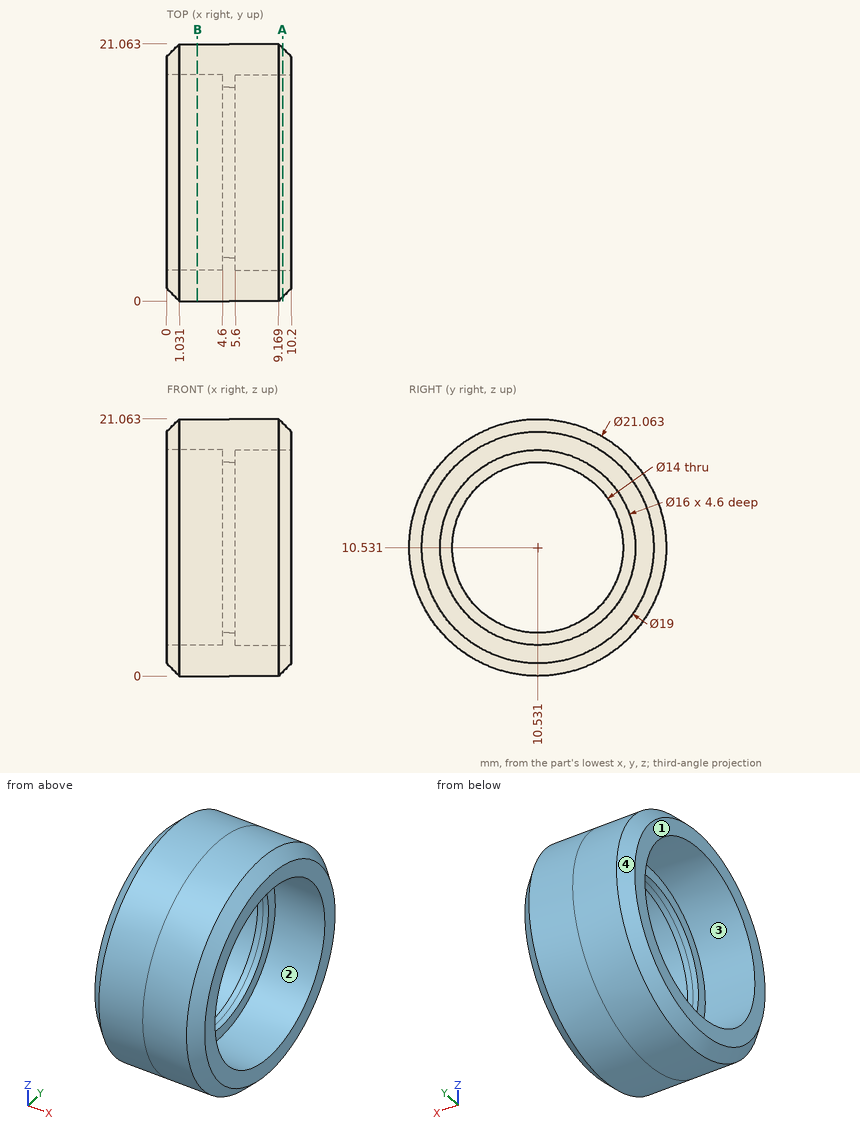
Input: dimensioned drawing with shaded views. Units: mm. Origin: part minimum x, y, z. Coordinates: 2 decimals unless noted, no trailing zeros. Order: outer loops, then holes, each group sorted by start corner. A loop starts at its lowest first (then second) coordinate and runs counter-clockwise, first axis right, second up.
1. Contact query for flat-ended pins moving along their axis: P1, Ø11, axis at y = 10.53, z = 10.53, coming from the -X side; P2, Ø8, axis at y = 12.5, z = 13.5, coming from the -X side; P3, Ø5, axis at x = 3, y = 15, coming from the +Z side; P4, Ø4, axis at x = 6.5, y = 4, coming from the +Z side. Output: stop coordinate, or through.
Checked values:
P1: passes through
P2: stops at x = 4.6
P3: stops at z = 20.88
P4: stops at z = 20.04
2. Cut plane A-A, the plane x = 9.5. Return loops of the section in (y, z), plus the area to 3 significant figures.
Checked values:
outline: circle Ø20.4 at (10.53, 10.53); hole circle Ø16 at (10.53, 10.53)
area: 126 mm2
3. Ray query, line 1 along Z through (x, y) = (3.75, 8.25); line 2 along Z through (x, y) = (3.25, 5.75) (1 decimal); line 3 along X through (y, z) = (16.5, 15.25). Return the intervals inside material, ascending.
Checked values:
line 1: z = 0.25 to 2.86, 18.2 to 20.81
line 2: z = 1.1 to 4.1, 16.9 to 19.9
line 3: x = 4.6 to 5.6
4. Draft query along Z for the marked faces 1, 2, 3 and 4. Return one class per face: +Z half, -Z half, draft (parallel to the pull), parting line (faces both ways), or undercut.
Checked values:
face 1: draft
face 2: undercut
face 3: undercut
face 4: parting line
5. Cut plane B-B, the plane x = 2.5. Return loops of the section in (y, z), plus the area to 3 significant figures.
Checked values:
outline: circle Ø21.06 at (10.53, 10.53); hole circle Ø16 at (10.53, 10.53)
area: 147 mm2
